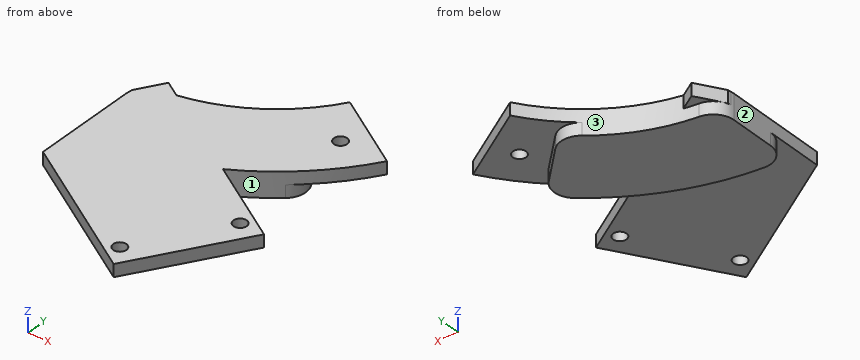
from build123d import *

# Parameters (mm, degrees)
EXTRUDE_1_DEPTH = 3
FILLET_1_R      = 5
SKETCH_2_R      = 1.6000000000000019
EXTRUDE_2_DEPTH = 3
FILLET_2_R      = 5
SKETCH_3_R      = 1.6000000000000008
SKETCH_3_R_2    = 1.6000000000000012
EXTRUDE_3_DEPTH = 3


with BuildPart() as part:
    # 草图1 → 凸台-拉伸1 (new body)
    with BuildSketch(Plane.XY):
        with BuildLine():
            Line((-20.304339314515776, -30.013405439405844), (-20.304339314515772, -51.013405439405844))
            ThreePointArc((-20.304339314515772, -51.013405439405844), (3.4220334921198514, -46.293936455105595), (23.536281119050262, -32.854025872971704))
            Line((23.536281119050262, -32.854025872971704), (8.687038714132733, -18.00478346805423))
            ThreePointArc((8.687038714132733, -18.00478346805423), (-4.614318587547064, -26.892466272368587), (-20.304339314515776, -30.013405439405844))
        make_face()
    extrude(amount=EXTRUDE_1_DEPTH)

    # 圆角1
    fillet_1_edges = [part.edges().sort_by_distance(p)[0] for p in [
        (8.687038714132733, -18.004783468054235, 1.5),
        (23.53628111905026, -32.854025872971704, 1.5),
        (-20.304339314515772, -51.013405439405844, 1.5),
        (-20.304339314515772, -30.013405439405844, 1.5),
    ]]
    fillet(fillet_1_edges, radius=FILLET_1_R)

    # 草图2 → 凸台-拉伸2 (add)
    with BuildSketch(Plane.XY.offset(3)):
        with BuildLine():
            Line((-20.30433931451578, -30.013405439405844), (-20.30433931451578, -51.013405439405865))
            ThreePointArc((-20.30433931451578, -51.013405439405865), (9.745319415064024, -43.24455894212779), (32.26429472639552, -21.884954156689382))
            Line((32.26429472639552, -21.884954156689382), (14.45878964802233, -10.751042494383663))
            ThreePointArc((14.45878964802233, -10.751042494383663), (-0.43279079979365775, -24.87594243314131), (-20.30433931451578, -30.013405439405844))
        make_face()
        with Locations((21.227676100740037, -22.06013948042292)):
            Circle(SKETCH_2_R, mode=Mode.SUBTRACT)
    extrude(amount=EXTRUDE_2_DEPTH)

    # 圆角2
    fillet_2_edges = [part.edges().sort_by_distance(p)[0] for p in [
        (-20.30433931451578, -30.013405439405844, 4.5),
        (-20.30433931451578, -51.01340543940586, 4.5),
    ]]
    fillet(fillet_2_edges, radius=FILLET_2_R)

    # 草图3 → 凸台-拉伸3 (add)
    with BuildSketch(Plane.XY.offset(6)):
        Polygon((-16.298731474091507, -26.90045671258201), (29.48685301315381, -55.53051527279668), (13.581264924145668, -80.96695109904408), (-20.30433931451578, -59.778036628128184), (-20.30433931451578, -34.74085890010055), (-20.159852559425826, -33.075214801052134), align=None)
        with Locations((-13.649884311951084, -32.09503164337476)):
            Circle(SKETCH_3_R, mode=Mode.SUBTRACT)
        with Locations((23.656888233211756, -55.42322750725339)):
            Circle(SKETCH_3_R, mode=Mode.SUBTRACT)
        with Locations((10.932417762005228, -75.7723761682513)):
            Circle(SKETCH_3_R_2, mode=Mode.SUBTRACT)
    extrude(amount=-EXTRUDE_3_DEPTH)


solid = part.part
Here's how the part is built. I have some questions about the finished solid (model axes, mm). Face numbers are marked on the shaded views. Give positions to 0.01 mm unless a question says otherwise; leave off trailing zeros. Order: outer loops, then holes, each group sorted by start corner. A loop starts at its lowest first (then second) coordinate and runs counter-clockwise, first axis right, second up. Notation, with made-up numbers: (32.25, 48) -> (68.25, 48) arc R21 ccw to (68.25, 81) -> close; hole circle Ø4 at (81.25, 3.25). An arc over 180 degrees is marked (long way). Use a Markdown table: item, result. Add a question column.
Item 1: I need wall thicknesses on line 1 (Y direction, x = 11.5, z = 3.2); line 2 (Z direction, x = -8.5, y = -60); line 3 (Y direction, x = 24.5, z = 4.7). Which ranges of each line are inside material? Lowest first, please.
Item 2: If we mould it in two halves opening along Y, with no side actions, what happens to the marked faces 1, 2 and 3? For each: pulls with the +Y half, pulls with the -Y half, needs draft (parallel to the pull), parting line crosses it, or undercut.
Item 3: Will these pins go through, and if not, where does the flat tip stop? pin 1 (1.5 mm diameter, centred on x = 9, z = 2, fed in from +Y); pin 2 (3 mm diameter, centred on x = 10.93, y = -75.77, fed in from -Z); pin 3 (3 mm diameter, centred on y = -71.5, z = 5, fed in from -X); pin 4 (2 mm diameter, centred on x = 17, z = 3, fed in from +Y).
Item 4: Imagine slicing it at C-C on x = -8.5. Please give me the cut outline in (y, z), plus the area to 3 significant figures.
Item 5: Imagine slicing it at A-A on z = 3.75. Please give me the cut outline in (x, y).
Item 6: Imagine slicing it at D-D on y = -66. Please give me the cut outline in (x, z).
Item 7: Imagine slicing it at B-B on y = -25.5. Please give me the cut outline in (x, z).
Data:
| question | item | result |
|---|---|---|
| 1 | line 1 | y = -79.67 to -77.27, -74.28 to -44.28, -42.23 to -14.89 |
| 1 | line 2 | z = 3 to 6 |
| 1 | line 3 | y = -63.51 to -56.78, -54.06 to -52.41, -31.87 to -17.03 |
| 2 | face 1 | undercut |
| 2 | face 2 | needs draft |
| 2 | face 3 | pulls with the +Y half |
| 3 | pin 1 | stops at y = -19.88 |
| 3 | pin 2 | passes through |
| 3 | pin 3 | stops at x = -3.96 |
| 3 | pin 4 | stops at y = -11.71 |
| 4 | outline | (-67.16, 3) -> (-49.88, 3) -> (-49.88, 0) -> (-28.28, 0) -> (-28.28, 6) -> (-67.16, 6) -> close |
| 4 | area | 181 mm² |
| 5 | outline | (-20.3, -59.78) -> (13.58, -80.97) -> (29.49, -55.53) -> (9.79, -43.22) arc R62 ccw to (32.26, -21.88) -> (14.46, -10.75) arc R41 cw to (-12.51, -29.27) -> (-16.3, -26.9) -> (-20.16, -33.08) -> (-20.23, -33.88) arc R5 ccw to (-20.3, -34.74) -> close; hole circle Ø3.2 at (10.93, -75.77); hole circle Ø3.2 at (21.23, -22.06); hole circle Ø3.2 at (23.66, -55.42) |
| 6 | outline | (-10.35, 3) -> (22.94, 3) -> (22.94, 6) -> (-10.35, 6) -> close |
| 7 | outline | (-1.6, 0) -> (16.18, 0) -> (16.18, 3) -> (29.82, 3) -> (29.82, 6) -> (-1.6, 6) -> close |
